Verification items for the finished model (mm, model axes). Give positions to 0.01 mm unless a question says otherwise; leave off trailing zeros. Loops run counter-clockwise (first coordinate to the right, second up) from the corner with the lowest first, then second, coordinate; pieces in that order, holes last. Notation, with made-up numbers: M 58,7 L 91,7 A17 ccw 91,18 Z; hole C 41.25,42 d11. An arc over 180 degrees is marked long. Use CSV: the item, a comma, the result in double quotes.
from build123d import *

# Parameters (mm, degrees)
F0_W     = 85.598
F0_H     = 127
F0_R     = 6.35
F0_R_2   = 36.957
F1_DEPTH = 4.7625
F3_DEPTH = 4.7635


with BuildPart() as f1:
    # F0 (on Right) → F1 (new body)
    with BuildSketch(Plane.YZ):
        Rectangle(F0_W, F0_H)
        with Locations((-22.5, -44)):
            Circle(F0_R, mode=Mode.SUBTRACT)
        with Locations((22.5, -44)):
            Circle(F0_R, mode=Mode.SUBTRACT)
        with Locations((-22.5, 44)):
            Circle(F0_R, mode=Mode.SUBTRACT)
        Circle(F0_R_2, mode=Mode.SUBTRACT)
        with Locations((22.5, 44)):
            Circle(F0_R, mode=Mode.SUBTRACT)
    extrude(amount=F1_DEPTH)

    # F2 (on Right) → F3 (cut, through all)
    with BuildSketch(Plane.YZ):
        with BuildLine():
            Line((-42.799, -31.75), (-42.799, -44.45))
            Line((-42.799, -44.45), (-40.256551, -44.45))
            ThreePointArc((-40.256551, -44.45), (-37.856895, -44.629605), (-38.0365, -42.229949))
            Line((-38.0365, -42.229949), (-38.0365, -33.970051))
            ThreePointArc((-38.0365, -33.970051), (-37.856895, -31.570395), (-40.256551, -31.75))
            Line((-40.256551, -31.75), (-42.799, -31.75))
        make_face()
        with BuildLine():
            Line((42.799, -44.45), (42.799, -31.75))
            Line((42.799, -31.75), (40.256551, -31.75))
            ThreePointArc((40.256551, -31.75), (37.856895, -31.570395), (38.0365, -33.970051))
            Line((38.0365, -33.970051), (38.0365, -42.229949))
            ThreePointArc((38.0365, -42.229949), (37.856895, -44.629605), (40.256551, -44.45))
            Line((40.256551, -44.45), (42.799, -44.45))
        make_face()
    extrude(amount=F3_DEPTH, mode=Mode.SUBTRACT)


solid = f1.part
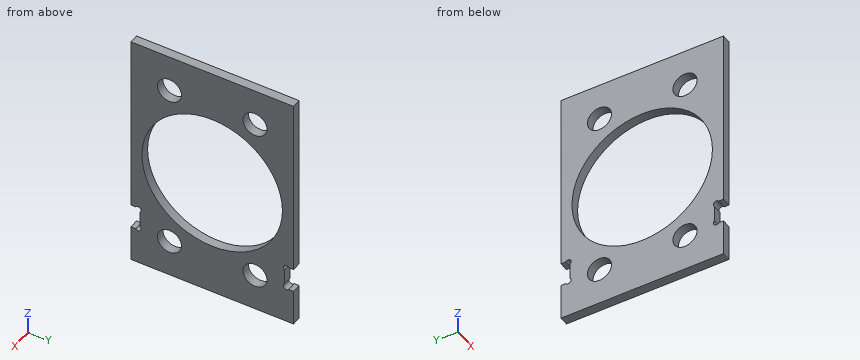
(1) Section check D-D on y = -7.5. Record the cut outline in (x, z).
Calculated:
outline,"M 0,-63.5 L 4.76,-63.5 L 4.76,-36.19 L 0,-36.19 Z; M 0,36.19 L 4.76,36.19 L 4.76,63.5 L 0,63.5 Z"
(2) Section check A-A on z = 0. Record the cut outline in (x, y), plus the area to 3 significant figures.
Calculated:
outline,"M 0,-42.8 L 4.76,-42.8 L 4.76,-36.96 L 0,-36.96 Z; M 0,36.96 L 4.76,36.96 L 4.76,42.8 L 0,42.8 Z"
area,"55.6 mm²"
(3) Section check C-C on x = 3.95. Count the separate pieces of the cut face and the enclosed holes in it, plus the area to 3 significant figures.
Calculated:
separate pieces,"1"
enclosed holes,"5"
area,"5,940 mm²"
(4) Scan lines: L1, parallel to Z at x = 1.15, y = 38; L2, parallel to Y at x = 1.1, z = 40; L3, parallel to Z at x = 2.75, y = -22.5. Record each from-to range of solid material in increasing order. Write a range as from..to.
Calculated:
L1,"z = -63.5..-44.76, -42.26..-33.94, -31.44..63.5"
L2,"y = -42.8..-27.43, -17.57..17.57, 27.43..42.8"
L3,"z = -63.5..-50.35, -37.65..-29.32, 29.32..37.65, 50.35..63.5"
(5) Depth check by flat-ended pin: pin 1 Ø7.5 at (y, z) = (22.5, 44) entering from -X. Enter the tip coordinate at first touch or a pass-through.
Calculated:
pin 1,"passes through"
(6) Section check B-B on z = 44. Record the cut outline in (x, y).
Calculated:
outline,"M 0,-42.8 L 4.76,-42.8 L 4.76,-28.85 L 0,-28.85 Z; M 0,-16.15 L 4.76,-16.15 L 4.76,16.15 L 0,16.15 Z; M 0,28.85 L 4.76,28.85 L 4.76,42.8 L 0,42.8 Z"
